from build123d import *
from OCP.BRepFilletAPI import BRepFilletAPI_MakeChamfer

# Parameters (mm, degrees)
ESQUISSE1_W             = 100
ESQUISSE1_H             = 10
BOSS_EXTRU_1_DEPTH      = 8
ESQUISSE2_W             = 100
ESQUISSE2_H             = 47.5
BOSS_EXTRU_2_DEPTH      = 10
BOSS_EXTRU_3_START      = -18
ESQUISSE3_R             = 2.75
BOSS_EXTRU_3_DEPTH      = 18
CONG_1_R                = 6
ESQUISSE5_W             = 100
ESQUISSE5_H             = 47.5
ENL_V_MAT_EXTRU_2_DEPTH = 3
ESQUISSE6_R             = 2.75
ENL_V_MAT_EXTRU_3_DEPTH = 225.162887353
ESQUISSE7_W             = 60
ESQUISSE7_H             = 60
BOSS_EXTRU_4_DEPTH      = 5
CONG_2_R                = 10
CHANFREIN2_SIZE         = 3
ESQUISSE8_R             = 1.5
ENL_V_MAT_EXTRU_4_DEPTH = 224.81688959
BOSS_EXTRUDE1_DEPTH     = 18
BOSS_EXTRUDE2_DEPTH     = 5
SKETCH6_R               = 2
CUT_EXTRUDE3_DEPTH      = 15
CUT_EXTRUDE2_DEPTH      = 18
MIRROR4_COPY_1_DEPTH    = 5
BOSS_EXTRUDE3_START     = 5
BOSS_EXTRUDE3_DEPTH     = 5
CHAMFER1_SIZE           = 28.356409098
CHAMFER1_SIZE_2         = 5
CHAMFER2_SIZE           = 5
FILLET2_R               = 5
FILLET1_R               = 5


# Some blends are built 0.0001 mm under size
with BuildPart() as part:
    # Esquisse1 → Boss.-Extru.1 (new body)
    with BuildSketch(Plane.XY):
        with BuildLine():
            Line((0, 0), (120, 0))
            Line((120, 0), (120, 70))
            Line((120, 70), (135, 130))
            ThreePointArc((135, 130), (60, 170), (-15, 130))
            Line((-15, 130), (0, 70))
            Line((0, 70), (0, 0))
        make_face()
        with Locations((60, 55)):
            Rectangle(ESQUISSE1_W, ESQUISSE1_H, mode=Mode.SUBTRACT)
        with Locations((60, 29.5)):
            Rectangle(ESQUISSE1_W, ESQUISSE1_H, mode=Mode.SUBTRACT)
        with BuildLine():
            Line((8, 70), (-6.536529961, 128.146119843))
            ThreePointArc((-6.536529961, 128.146119843), (60, 162), (126.536529961, 128.146119843))
            Line((126.536529961, 128.146119843), (112, 70))
            Line((112, 70), (8, 70))
        make_face(mode=Mode.SUBTRACT)
    extrude(amount=BOSS_EXTRU_1_DEPTH)

    # Esquisse2 → Boss.-Extru.2 (add)
    with BuildSketch(Plane.XY.offset(8)):
        with BuildLine():
            Line((0, 70), (0, 0))
            Line((0, 0), (120, 0))
            Line((120, 0), (120, 70))
            Line((120, 70), (135, 130))
            ThreePointArc((135, 130), (60, 170), (-15, 130))
            Line((-15, 130), (0, 70))
        make_face()
        with Locations((60, 42.25)):
            Rectangle(ESQUISSE2_W, ESQUISSE2_H, mode=Mode.SUBTRACT)
        with BuildLine():
            Line((112, 70), (126.536529961, 128.146119843))
            ThreePointArc((126.536529961, 128.146119843), (60, 162), (-6.536529961, 128.146119843))
            Line((-6.536529961, 128.146119843), (8, 70))
            Line((8, 70), (112, 70))
        make_face(mode=Mode.SUBTRACT)
    extrude(amount=BOSS_EXTRU_2_DEPTH)

    # Esquisse3 → Boss.-Extru.3 (add)
    # profile 1 of 2: a face of its own
    with BuildSketch(Plane.XY.offset(18).offset(BOSS_EXTRU_3_START)):
        with BuildLine():
            Line((0, 47), (0, 54))
            Line((0, 54), (-13, 54))
            Line((-13, 54), (-13, -12))
            ThreePointArc((-13, -12), (-3, -22), (7, -12))
            Line((7, -12), (7, 0))
            Line((7, 0), (0, 0))
            Line((0, 0), (0, 7))
            Line((0, 7), (-6, 7))
            Line((-6, 7), (-6, 47))
            Line((-6, 47), (0, 47))
        make_face()
        with Locations((-3, -12)):
            Circle(ESQUISSE3_R, mode=Mode.SUBTRACT)
    # profile 2 of 2: a face of its own
    with BuildSketch(Plane.XY.offset(18).offset(BOSS_EXTRU_3_START)):
        with BuildLine():
            Line((-5.941176471, 125.764705882), (-6.536529961, 128.146119843))
            ThreePointArc((-6.536529961, 128.146119843), (-5.777042038, 129.172127886), (-5.001734316, 130.18623456))
            ThreePointArc((-5.001734316, 130.18623456), (-24.781648189, 132.078306694), (-5.941176471, 125.764705882))
        make_face()
    boss_extru_3 = extrude(amount=BOSS_EXTRU_3_DEPTH)

    # Symétrie1: Boss.-Extru.3 across plane
    add(boss_extru_3.mirror(Plane.ZY.offset(-60)))

    # Congé1
    cong_1_edges = [part.edges().sort_by_distance(p)[0] for p in [
        (7, 0, 9),
        (0, 54, 9),
        (-13, 54, 9),
        (-8.977845414, 137.983336029, 9),
        (-12.57464375, 120.298574999, 9),
        (133, 54, 9),
        (113, 0, 9),
        (120, 54, 9),
        (132.57464375, 120.298574999, 9),
        (128.977845414, 137.983336029, 9),
    ]]
    fillet(cong_1_edges, radius=CONG_1_R)

    # Esquisse5 → Enlèv. mat.-Extru.2 (cut)
    with BuildSketch(Plane.XY.offset(8)):
        with Locations((60, 42.25)):
            Rectangle(ESQUISSE5_W, ESQUISSE5_H)
    extrude(amount=-ENL_V_MAT_EXTRU_2_DEPTH, mode=Mode.SUBTRACT)

    # Esquisse6 → Enlèv. mat.-Extru.3 (cut, through all)
    with BuildSketch(Plane.XY.offset(18)):
        with Locations((-15, 130)):
            Circle(ESQUISSE6_R)
        with Locations((135, 130)):
            Circle(ESQUISSE6_R)
    extrude(amount=-ENL_V_MAT_EXTRU_3_DEPTH, mode=Mode.SUBTRACT)

    # Esquisse7 → Boss.-Extru.4 (add)
    with BuildSketch(Plane(origin=(0, 0, 0), x_dir=(-1, 0, 0), z_dir=(0, 0, -1))):
        with Locations((-60, -30)):
            Rectangle(ESQUISSE7_W, ESQUISSE7_H)
    extrude(amount=-BOSS_EXTRU_4_DEPTH)

    # Congé2
    cong_2_edges = [part.edges().sort_by_distance(p)[0] for p in [
        (60, 0, 5),
        (90, 0, 2.5),
        (30, 0, 2.5),
    ]]
    fillet(cong_2_edges, radius=CONG_2_R)

    # Chanfrein2
    chanfrein2_edges = [part.edges().sort_by_distance(p)[0] for p in [
        (-5.75, -12, 18),
        (125.75, -12, 18),
        (-17.75, 130, 18),
        (132.25, 130, 18),
    ]]
    chamfer(chanfrein2_edges, length=CHANFREIN2_SIZE)

    # Esquisse8 → Enlèv. mat.-Extru.4 (cut, through all)
    with BuildSketch(Plane.XY.offset(5)):
        with Locations((40, -43.333333333)):
            Circle(ESQUISSE8_R)
        with Locations((40, -26.666666667)):
            Circle(ESQUISSE8_R)
        with Locations((60, -26.666666667)):
            Circle(ESQUISSE8_R)
        with Locations((60, -43.333333333)):
            Circle(ESQUISSE8_R)
        with Locations((80, -26.666666667)):
            Circle(ESQUISSE8_R)
        with Locations((80, -43.333333333)):
            Circle(ESQUISSE8_R)
    extrude(amount=-ENL_V_MAT_EXTRU_4_DEPTH, mode=Mode.SUBTRACT)

    # Sketch2 → Boss-Extrude1 (add)
    with BuildSketch(Plane.XY.offset(18)):
        with BuildLine():
            Line((-8, 60), (-8, 102))
            Line((-8, 102), (0, 70))
            Line((0, 70), (0, 60))
            ThreePointArc((0, 60), (-3.283009434, 56.352815094), (-8, 55))
            Line((-8, 55), (-8, 60))
        make_face()
    boss_extrude1 = extrude(amount=-BOSS_EXTRUDE1_DEPTH)

    # Sketch3 → Boss-Extrude2 (add)
    with BuildSketch(Plane(origin=(0, 0, 0), x_dir=(-1, 0, 0), z_dir=(0, 0, -1))):
        Polygon((8, 102), (8, 47), (-10, 47), (-10, 70), (-8, 70), (0, 102), align=None)
    boss_extrude2 = extrude(amount=BOSS_EXTRUDE2_DEPTH)

    # Sketch6 → Cut-Extrude3 (cut)
    with BuildSketch(Plane.ZY.offset(8)):
        with Locations(Location((9, 65, 0), (0, 0, 270))):
            Circle(SKETCH6_R)
    cut_extrude3 = extrude(amount=-CUT_EXTRUDE3_DEPTH, mode=Mode.SUBTRACT)

    # Mirror1: Boss-Extrude1, Cut-Extrude3 across plane
    add(boss_extrude1.mirror(Plane.ZY.offset(-60)))
    add(cut_extrude3.mirror(Plane.ZY.offset(-60)), mode=Mode.SUBTRACT)

    # Mirror3: Boss-Extrude2 across plane
    add(boss_extrude2.mirror(Plane.ZY.offset(-60)))

    # Sketch4 → Cut-Extrude2 (cut)
    with BuildSketch(Plane.XY.offset(18)):
        with BuildLine():
            Line((120, 70), (0, 70))
            Line((0, 70), (0, 60))
            ThreePointArc((0, 60), (-1.757359313, 55.757359313), (-6, 54))
            Line((-6, 54), (-7, 54))
            ThreePointArc((-7, 54), (-11.242640687, 52.242640687), (-13, 48))
            Line((-13, 48), (-13, -60))
            Line((-13, -60), (133, -60))
            Line((133, -60), (133, 48))
            ThreePointArc((133, 48), (131.242640687, 52.242640687), (127, 54))
            Line((127, 54), (126, 54))
            ThreePointArc((126, 54), (121.757359313, 55.757359313), (120, 60))
            Line((120, 60), (120, 70))
        make_face()
    extrude(amount=-CUT_EXTRUDE2_DEPTH, mode=Mode.SUBTRACT)

    # Mirror4: Boss-Extrude2 across plane
    add(boss_extrude2.mirror(Plane.XY.offset(9)))

    # Mirror4 copy 1 sketch → Mirror4 copy 1 (add)
    with BuildSketch(Plane(origin=(120, 0, 18), x_dir=(1, 0, 0), z_dir=(0, 0, 1))):
        Polygon((8, 102), (8, 47), (-10, 47), (-10, 70), (-8, 70), (0, 102), align=None)
    extrude(amount=MIRROR4_COPY_1_DEPTH)

    # Sketch5 → Boss-Extrude3 (add)
    with BuildSketch(Plane(origin=(0, 0, 0), x_dir=(-1, 0, 0), z_dir=(0, 0, -1)).offset(BOSS_EXTRUDE3_START)):
        with BuildLine():
            Line((-131.402615329, 115.610461316), (-128, 102))
            Line((-128, 102), (-120, 102))
            Line((-120, 102), (-125.941176471, 125.764705882))
            ThreePointArc((-125.941176471, 125.764705882), (-130.2319164, 121.209927259), (-136.389668956, 120.097029729))
            ThreePointArc((-136.389668956, 120.097029729), (-133.210561548, 118.615803933), (-131.402615329, 115.610461316))
        make_face()
        with BuildLine():
            ThreePointArc((-126.075357318, 141.25368237), (-128.884007473, 139.55597192), (-132.165711776, 139.589932756))
            ThreePointArc((-132.165711776, 139.589932756), (-127.045379023, 136.060033425), (-125.001734316, 130.18623456))
            ThreePointArc((-125.001734316, 130.18623456), (-60, 162), (5.001734316, 130.18623456))
            ThreePointArc((5.001734316, 130.18623456), (7.045379023, 136.060033425), (12.165711776, 139.589932756))
            ThreePointArc((12.165711776, 139.589932756), (8.884007473, 139.55597192), (6.075357318, 141.25368237))
            ThreePointArc((6.075357318, 141.25368237), (-60, 170), (-126.075357318, 141.25368237))
        make_face()
        with BuildLine():
            ThreePointArc((16.389668956, 120.097029729), (10.2319164, 121.209927259), (5.941176471, 125.764705882))
            Line((5.941176471, 125.764705882), (0, 102))
            Line((0, 102), (8, 102))
            Line((8, 102), (11.402615329, 115.610461316))
            ThreePointArc((11.402615329, 115.610461316), (13.210561548, 118.615803933), (16.389668956, 120.097029729))
        make_face()
    extrude(amount=-BOSS_EXTRUDE3_DEPTH)

    # Chamfer1
    chamfer1_edges_1 = [part.edges().sort_by_distance(p)[0] for p in [
        (124, 102, 23),
    ]]
    chamfer1_side_1 = [part.faces().sort_by_distance(p)[0] for p in [
        (124, 101.9, 23),
    ]]
    chamfer1_edges_2 = [part.edges().sort_by_distance(p)[0] for p in [
        (-4, 102, 23),
    ]]
    chamfer1_side_2 = [part.faces().sort_by_distance(p)[0] for p in [
        (-4, 102, 22.9),
    ]]
    chamfer1 = BRepFilletAPI_MakeChamfer(part.part.solid().wrapped)
    for e in chamfer1_edges_1:
        chamfer1.Add(CHAMFER1_SIZE - 0.0001, CHAMFER1_SIZE_2 - 0.0001, e.wrapped, chamfer1_side_1[0].wrapped)
    for e in chamfer1_edges_2:
        chamfer1.Add(CHAMFER1_SIZE_2 - 0.0001, CHAMFER1_SIZE - 0.0001, e.wrapped, chamfer1_side_2[0].wrapped)
    add(Compound.cast(chamfer1.Shape()), mode=Mode.REPLACE)  # a hair under: the kernel refuses the full size

    # Chamfer2
    chamfer2_edges = [part.edges().sort_by_distance(p)[0] for p in [
        (130.2319164, 121.209927259, -5),
        (-7.045379023, 136.060033425, -5),
        (127.045379023, 136.060033425, -5),
        (-10.2319164, 121.209927259, -5),
    ]]
    chamfer(chamfer2_edges, length=CHAMFER2_SIZE - 0.0001)  # a hair under: the kernel refuses the full size

    # Fillet2
    # the kernel refuses this fillet: 5 mm, written as the material it adds along each edge
    with BuildSketch(Plane(origin=(8, 70, -5), x_dir=(-0.2425356250363325, 0.970142500145332, 0), z_dir=(0, 0, 1)), Plane(origin=(8, 70, 18), x_dir=(-0.2425356250363325, 0.970142500145332, 0), z_dir=(0, 0, 1))) as fillet2_piece_1:
        with BuildLine():
            CenterArc((3.46943809, -5), FILLET2_R, 90, 52.269872505)
            Line((-0.48507125, -1.940285), (0, 0))
            Line((0, 0), (3.46943809, 0))
        make_face()
    extrude(amount=5)
    with BuildSketch(Plane(origin=(112, 70, -5), x_dir=(0.2425356250363291, 0.9701425001453328, 0), z_dir=(0, 0, 1)), Plane(origin=(112, 70, 18), x_dir=(0.2425356250363291, 0.9701425001453328, 0), z_dir=(0, 0, 1))) as fillet2_piece_2:
        with BuildLine():
            CenterArc((3.46943809, 5), FILLET2_R, 217.730127495, 52.269872505)
            Line((-0.48507125, 1.940285), (0, 0))
            Line((0, 0), (3.46943809, 0))
        make_face()
    extrude(amount=5)

    # Fillet1
    fillet1_edges = [part.edges().sort_by_distance(p)[0] for p in [
        (110, 58.5, 23),
        (10, 58.5, 23),
        (1, 47, 23),
        (119, 47, 23),
    ]]
    fillet(fillet1_edges, radius=FILLET1_R - 0.0001)  # a hair under: the kernel refuses the full size


solid = part.part
Geometry check sheet. Reference: the model listing, model coordinates, mm. A direction names the side the tool comes from. Give positions to 0.01 mm unless a question says otherwise; leave off trailing zeros. Loops run counter-clockwise (first coordinate to the right, second up) from the corner with the lowest first, then second, coordinate; pieces in that order, holes last. Notation, with made-up numbers: (13.25, 16) -> (51.25, 16) arc R22 ccw to (51.25, 37) -> close; hole circle Ø11 at (-19, -33.5). An arc over 180 degrees is marked (long way). Answer in a Markdown table with one row per item. Add a question column.
1) Cross-section at D-D on y = 105.5. Record the boundary of the cut face in (x, z) (3 decimals), and give its area (3 significant figures).
2) Material ranges on probe 1 along X at (y, z) = (69, 14); probe 2 along Z at (x, y) = (123, 65); probe 3 along X at (y, z) = (86.5, 3) (3 decimals), recorded low to high. Write a range as from..to.
3) Cross-section at B-B on y = 80.5. Record the boundary of the cut face in (x, z) (3 decimals).
4) Cross-section at C-C on x = 26.5. Record the boundary of the cut face in (y, z).
5) Draft check along Y on faces 1 (the face through (8.168, 71.378, -2.535)), 2 (the face through (7.864, 71.783, 19.722)), 3 (the face through (123.224, 56.39, 9.126)), 4 (the face through (-17.893, 130.127, 15.146)). Enter one of: pulls with the +Y half, pulls with the -Y half, needs draft (parallel to the pull), parting line crosses it, or undercut.
6) Cross-section at A-A on z = 9. State how many separate pieces and enclosed holes the cut face has, and give its area (3 significant figures).
7) Set-up check for faces 5 (the face through (111.79, 71.33, -2.54)), 6 (the face through (128, 75, 9)), 7 (the face through (116, 70, 9)), 8 (the face through (112.1, 71.73, 19.72)): record each of +Z, -Z, +X, -X, +Y, -Y from which the full face is reachable in a straight line by a thin tool's end or side.
8) Gauge pin test, flat ends, axial feed: P1, Ø5, axis at y = 125, z = 3, coming from the +X side; P2, Ø5.5, axis at y = 62.5, z = -3, coming from the -X side; P3, Ø5, axis at y = 64, z = 9, coming from the +X side; P4, Ø20.5, axis at x = 85.5, y = 145, coming from the +Z side. Record the tip position at first contact, or that the pin passes through.
Outcome:
| question | item | result |
|---|---|---|
| 1 | outline | (-8.875, -5) -> (-0.875, -5) -> (-0.875, 18) -> (-8.875, 18) -> close; (120.875, -5) -> (128.875, -5) -> (128.875, 18) -> (120.875, 18) -> close |
| 1 | area | 368 mm^2 |
| 2 | probe 1 | x = -8..0, 120..128 |
| 2 | probe 2 | z = -5..7, 11..23 |
| 2 | probe 3 | x = -8..3.875, 116.125..128 |
| 3 | outline | (-8, -5) -> (5.375, -5) -> (5.375, 21.791) -> (-8, 21.791) -> close; (114.625, -5) -> (128, -5) -> (128, 21.791) -> (114.625, 21.791) -> close |
| 4 | outline | (154.87, -5) -> (163.56, -5) -> (163.56, 18) -> (154.87, 18) -> close |
| 5 | face 1 | undercut |
| 5 | face 2 | pulls with the +Y half |
| 5 | face 3 | pulls with the -Y half |
| 5 | face 4 | undercut |
| 6 | separate pieces | 3 |
| 6 | enclosed holes | 2 |
| 6 | area | 3,050 mm^2 |
| 7 | face 5 | +Z, -Z |
| 7 | face 6 | +Z, -Z, +X, -Y |
| 7 | face 7 | -Y |
| 7 | face 8 | +Z, -Z, +Y |
| 8 | P1 | stops at x = 144.68 |
| 8 | P2 | stops at x = -8 |
| 8 | P3 | stops at x = 128 |
| 8 | P4 | passes through |
